The model under review builds one solid part; all positions refer to its coordinate system, in mm. A direction names the side the tool comes from. Round coordinates to 2 decimals unless told otherwise and drop trailing zeros. Order: outer loops, then holes, each group sorted by start corner. A loop starts at its lowest first (then second) coordinate and runs counter-clockwise, first axis right, second up.
```python
from build123d import *

# Parameters (mm, degrees)
F3_DEPTH = 31.75
F4_R     = 3.302
F5_DEPTH = 12.7
F6_DEPTH = 6.35


with BuildPart() as f3:
    # F2 (on Top) → F3 (new body)
    with BuildSketch(Plane.XY):
        with BuildLine():
            Line((24.45, -48.5775), (24.45, 48.5775))
            Line((24.45, 48.5775), (11.75, 48.5775))
            Line((11.75, 48.5775), (11.75, 24.4475))
            Line((11.75, 24.4475), (12.225, 0))
            ThreePointArc((12.225, 0), (0, -12.225), (-12.225, 0))
            ThreePointArc((-12.225, 0), (-15.1625, 2.9375), (-18.1, 0))
            ThreePointArc((-18.1, 0), (-15.0471149103, -10.0595393968), (-6.9183057596, -16.7256403589))
            Line((-6.9183057596, -16.7256403589), (11.75, -24.4475))
            Line((11.75, -24.4475), (11.75, -48.5775))
            Line((11.75, -48.5775), (24.45, -48.5775))
        make_face()
    extrude(amount=F3_DEPTH)

    # F4 (on face) → F5 (cut, through all)
    with BuildSketch(Plane(origin=(11.75, 0, 0), x_dir=(0, -1, 0), z_dir=(-1, 0, 0))):
        with Locations((-36.5125, 15.875)):
            Circle(F4_R)
        with Locations((36.5125, 15.875)):
            Circle(F4_R)
    extrude(amount=-F5_DEPTH, mode=Mode.SUBTRACT)

    # F4 (on face) → F6 (cut)
    with BuildSketch(Plane(origin=(11.75, 0, 0), x_dir=(0, -1, 0), z_dir=(-1, 0, 0))):
        Polygon((-30.7975, 12.5754432116), (-30.7975, 19.1745567884), (-36.5125, 22.4741135768), (-42.2275, 19.1745567884), (-42.2275, 12.5754432116), (-36.5125, 9.2758864232), align=None)
        with Locations((-36.5125, 15.875)):
            Circle(F4_R, mode=Mode.SUBTRACT)
        Polygon((30.7975, 19.1745567884), (30.7975, 12.5754432116), (36.5125, 9.2758864232), (42.2275, 12.5754432116), (42.2275, 19.1745567884), (36.5125, 22.4741135768), align=None)
        with Locations((36.5125, 15.875)):
            Circle(F4_R, mode=Mode.SUBTRACT)
    extrude(amount=-F6_DEPTH, mode=Mode.SUBTRACT)


solid = f3.part
```
(1) Consider section A-A (z = 13.5). State how many separate pieces and enclosed holes the cut face has, and give its area (3 significant figures).
Data:
separate pieces: 3
enclosed holes: 0
area: 1,320 mm2
(2) Consider section B-B (y = -2). Write out the cut boundary in (x, z), and give its area (3 significant figures).
Data:
outline: (-17.99, 0) - (-12.06, 0) - (-12.06, 31.75) - (-17.99, 31.75) - close; (12.06, 0) - (24.45, 0) - (24.45, 31.75) - (12.06, 31.75) - close
area: 582 mm2
(3) Insertion check: pin 1 (8.5 mm diameter, centred on y = -36.51, z = 15.88, fed in from -X); pin 2 (12 mm diameter, centred on y = 34.5, z = 18.5, fed in from -X); pin 3 (12 mm diameter, centred on x = -6, z = 10.5, fed in from -Y). Each pin has a flat end and moves straight along its axis. Give the tip position at first contact, or say it passes through.
Data:
pin 1: stops at x = 18.1
pin 2: stops at x = 11.75
pin 3: stops at y = -19.59
(4) For faces 1 (the flat face through (11.75, 42, 12)), 2 (the flat face through (11.75, -42, 12)), 3 (the flat face through (14.88, -39.41, 20.8)), list the 3-axis set-ups (+Z, -Z, +X, -X, +Y, -Y) from which the entire face can be reached by the end or side of a thin tool; tool diameter is ignored.
Data:
face 1: +Z, -Z, -X, +Y
face 2: +Z, -Z, -X, -Y
face 3: -X
(5) To check wall thickness, follow probe 1 along Y at (x, z) = (19.5, 16); probe 2 along X at (y, z) = (29, 11.5); probe 3 along X at (y, z) = (0.5, 27). State the ranges of each line that lie inside material, in increasing order.
Data:
probe 1: y = -48.58 to -39.81, -33.21 to 33.21, 39.81 to 48.58
probe 2: x = 11.75 to 24.45
probe 3: x = -18.06 to -12.27, 12.22 to 24.45
(6) Consider section D-D (x = -11). Write out the cut boundary in (y, z), and give its area (3 significant figures).
Data:
outline: (-14.37, 0) - (-5.33, 0) - (-5.33, 31.75) - (-14.37, 31.75) - close
area: 287 mm2
(7) Consider section C-C (y = 29.5). Write out the cut boundary in (x, z).
Data:
outline: (11.75, 0) - (24.45, 0) - (24.45, 31.75) - (11.75, 31.75) - close
(8) Draft analysis for pull direction Z (two halves, no side actions). For faces 4 (the flat face through (14.88, -33.7, 20.85)), 5 (the flat face through (17, 1, 0)), 6 (the flat face through (17, 1, 31.75)), 7 (the flat face through (24.45, -1, 16)), state which applies: pulls with the +Z half, pulls with the -Z half, needs draft (parallel to the pull), parting line crosses it, or undercut.
Data:
face 4: undercut
face 5: pulls with the -Z half
face 6: pulls with the +Z half
face 7: needs draft
